Can you work these out from the model? Positions are in its coordinate system, mm. A direction names the side the tool comes from. Round coordinates to 2 decimals unless told otherwise and drop trailing zeros. Write each loop counter-clockwise with the first axis right and the second up, starting at its lowest first coordinate (ties: lowest second). Pieces come first, ordered by that corner, then holes.
Q1. If we section it at B-B (y = 1.25): Please give me the cut outline in (x, z).
Q2. For faces 1 (the flat face through (0.625, 1, -12)), 2 (the flat face through (0.625, 1, 12)), 3 (the flat face through (-17, 1, 7.5)), which set-ups out of +Z, -Z, +X, -X, +Y, -Y let a thin tool reach every point of the face, with its end or its side?
Q3. If we section it at A-A (z = 0): Please give me the cut outline in (x, y), plus the area to 3 significant figures.
Q4. We'd pull the mould along Z, two halves only. Please class faces 4 (the flat face through (-21.555, 1, -13)), 5 (the cylindrical face through (-9.74, 3.18, 2.43)), 6 (the flat face through (-18, 1, -7.5)): +Z half, -Z half, draft (parallel to the pull), parting line (faces both ways), or undercut.
Q5. If we section it at C-C (x = 12): Please give me the cut outline in (y, z).
Q6. Please list where these lines run through material, in increasing order: line 1 along Y through (x, z) = (0, -8.5); line 2 along Z through (x, y) = (-17.5, 0.25); line 3 along X through (y, z) = (1.35, -12.5).
Q7. If we section it at D-D (z = 7): Please give me the cut outline in (x, y).
Q8. I'm going to push flat-ended pins straight in: pin 1 Ø5 at (x, z) = (5.5, -12.5) entering from +Y; pin 2 Ø1 at (x, z) = (-0.5, 5.5) entering from -Y; pin 3 Ø1.6 at (x, y) = (8.5, 1) entering from -Z; pin 4 Ø2 at (y, z) = (1.5, 1.5) entering from -X. Where does each tip first touch, or does it pass through?
from build123d import *

# Parameters (mm, degrees)
BOSS_EXTRUDE1_DEPTH = 2
SKETCH2_R           = 4
BOSS_EXTRUDE2_DEPTH = 2.4


with BuildPart() as part:
    # Sketch1 → Boss-Extrude1 (new body)
    with BuildSketch(Plane(origin=(0, 0, 0), x_dir=(1, 0, 0), z_dir=(0, 1, 0))):
        Polygon((0.624790047, 6.5), (0.624790047, 17.5), (-9.416796267, 17.5), (-21.555209953, 17.5), (-21.555209953, 7.5), (-13.555209953, 7.5), (-13.555209953, -7.5), (-21.555209953, -7.5), (-21.555209953, -17.5), (-9.416796267, -17.5), (0.624790047, -17.5), (0.624790047, -6.5), (14.624790047, -6.5), (14.624790047, 6.5), align=None)
    extrude(amount=BOSS_EXTRUDE1_DEPTH)

    # Sketch2 → Boss-Extrude2 (add)
    with BuildSketch(Plane(origin=(0, 2, 0), x_dir=(1, 0, 0), z_dir=(0, 1, 0))):
        with Locations((-6.563909953, 0)):
            Circle(SKETCH2_R)
    extrude(amount=BOSS_EXTRUDE2_DEPTH)


solid = part.part
A:
1. outline: (-21.56, -17.5) - (0.62, -17.5) - (0.62, -6.5) - (14.62, -6.5) - (14.62, 6.5) - (0.62, 6.5) - (0.62, 17.5) - (-21.56, 17.5) - (-21.56, 7.5) - (-13.56, 7.5) - (-13.56, -7.5) - (-21.56, -7.5) - close
2. face 1: -Z, +X, +Y, -Y
2. face 2: +Z, +X, +Y, -Y
2. face 3: -X, +Y, -Y
3. outline: (-13.56, 0) - (14.62, 0) - (14.62, 2) - (-2.56, 2) - (-2.56, 4.4) - (-10.56, 4.4) - (-10.56, 2) - (-13.56, 2) - close
3. area: 75.6 mm2
4. face 4: draft
4. face 5: parting line
4. face 6: undercut
5. outline: (0, -6.5) - (2, -6.5) - (2, 6.5) - (0, 6.5) - close
6. line 1: y = 0 to 2
6. line 2: z = -17.5 to -7.5, 7.5 to 17.5
6. line 3: x = -21.56 to 0.62
7. outline: (-13.56, 0) - (0.62, 0) - (0.62, 2) - (-13.56, 2) - close
8. pin 1: passes through
8. pin 2: stops at y = 0
8. pin 3: stops at z = -6.5
8. pin 4: stops at x = -13.56
